For this review, take the finished solid that the model builds, in its own axes (mm). A direction names the side the tool comes from. Coordinates: 2 decimals unless noted, no trailing zeros. Write each loop counter-clockwise with the first axis right and the second up, starting at its lowest first coordinate (ties: lowest second). Pieces come first, ordered by that corner, then holes. Notation, with made-up numbers: (38.25, 73) - (71.25, 73) arc R33 cw to (71.25, 102) - close; hole circle Ø10 at (-31.75, -26.5). An arc over 180 degrees is marked (long way). Write each question's results on one line, items separated by ' | '.
from build123d import *

# Parameters (mm, degrees)
SKETCH_1_W          = 57
SKETCH_1_H          = 37
EXTRUDE_1_DEPTH     = 2
SKETCH_2_W          = 20
SKETCH_2_H          = 2
EXTRUDE_2_DEPTH     = 4
SKETCH_3_R          = 1.05
CUT_EXTRUDE_1_DEPTH = 4
CUT_EXTRUDE_2_DEPTH = 10
FILLET_1_R          = 1.5


with BuildPart() as part:
    # 草图1 → 凸台-拉伸1 (new body)
    with BuildSketch(Plane(origin=(0, 0, 0), x_dir=(1, 0, 0), z_dir=(0, 1, 0))):
        Rectangle(SKETCH_1_W, SKETCH_1_H)
    extrude(amount=EXTRUDE_1_DEPTH)

    # 草图2 → 凸台-拉伸2 (add)
    with BuildSketch(Plane.XY.offset(18.5)):
        with Locations((-3.3, 1)):
            Rectangle(SKETCH_2_W, SKETCH_2_H)
    extrude_2 = extrude(amount=EXTRUDE_2_DEPTH)

    # 镜向1: 凸台-拉伸2 across plane
    add(extrude_2.mirror(Plane.XY))

    # 草图3 → 切除-拉伸1 (cut)
    with BuildSketch(Plane(origin=(0, 2, 0), x_dir=(1, 0, 0), z_dir=(0, 1, 0))):
        with Locations((7.75, 18.5)):
            Circle(SKETCH_3_R)
        with Locations((-14.35, 18.5)):
            Circle(SKETCH_3_R)
        with Locations((-14.35, -18.5)):
            Circle(SKETCH_3_R)
        with Locations((7.75, -18.5)):
            Circle(SKETCH_3_R)
    extrude(amount=-CUT_EXTRUDE_1_DEPTH, mode=Mode.SUBTRACT)

    # 草图4 → 切除-拉伸2 (cut)
    with BuildSketch(Plane(origin=(0, 2, 0), x_dir=(1, 0, 0), z_dir=(0, 1, 0))):
        Polygon((-24.5, -14.5), (-1.963644752, -14.5), (-24.5, 12.175685803), align=None)
        Polygon((-22.536355248, 14.5), (-1.5, -10.400175599), (-1.5, 14.5), align=None)
        Polygon((1.5, 14.5), (1.5, -10.400175599), (22.536355248, 14.5), align=None)
        Polygon((24.5, 12.175685803), (1.963644752, -14.5), (24.5, -14.5), align=None)
    extrude(amount=-CUT_EXTRUDE_2_DEPTH, mode=Mode.SUBTRACT)

    # 圆角1
    fillet_1_edges = [part.edges().sort_by_distance(p)[0] for p in [
        (1.963644752, 1, 14.5),
        (24.5, 1, -12.175685803),
        (24.5, 1, 14.5),
        (-24.5, 1, -12.175685803),
        (-1.963644752, 1, 14.5),
        (-24.5, 1, 14.5),
        (28.5, 1, 18.5),
        (-28.5, 1, 18.5),
        (-28.5, 1, -18.5),
        (28.5, 1, -18.5),
        (-22.536355248, 1, -14.5),
        (-1.5, 1, -14.5),
        (-1.5, 1, 10.400175599),
        (1.5, 1, -14.5),
        (22.536355248, 1, -14.5),
        (1.5, 1, 10.400175599),
    ]]
    fillet(fillet_1_edges, radius=FILLET_1_R)


solid = part.part
Q1. Take a section at B-B on z = 3.5. State the section outline as (x, y) points, plus the area to 3 significant figures.
Results found:
outline: (-28.5, 0) - (-24.5, 0) - (-24.5, 2) - (-28.5, 2) - close; (-11.26, 0) - (-7.33, 0) - (-7.33, 2) - (-11.26, 2) - close; (-1.5, 0) - (1.5, 0) - (1.5, 2) - (-1.5, 2) - close; (7.33, 0) - (11.26, 0) - (11.26, 2) - (7.33, 2) - close; (24.5, 0) - (28.5, 0) - (28.5, 2) - (24.5, 2) - close | area: 37.7 mm2
Q2. Take a section at A-A on x = -12.5. State the section outline as (y, z) points, plus the area to 3 significant figures.
Results found:
outline: (0, -22.5) - (2, -22.5) - (2, -14.5) - (0, -14.5) - close; (0, -2.62) - (2, -2.62) - (2, 2.03) - (0, 2.03) - close; (0, 14.5) - (2, 14.5) - (2, 22.5) - (0, 22.5) - close | area: 41.3 mm2
Q3. For pin 1 (1 mm diameter, centred on x = -21, y = 1, fed in from -Z); pin 2 (0.6 mm diameter, centred on y = 1.5, z = -20, fed in from -X); pin 3 (1 mm diameter, centred on y = 1, z = 20, fed in from +X), all flat-tipped, find the tip position at first contact; note any pin that passes through.
Results found:
pin 1: z = -18.5 | pin 2: x = -13.3 | pin 3: x = 6.7
Q4. Wall thickness on line 1 along Z through (x, y) = (23, 0.9); line 2 along X through (y, z) = (1, -3); line 3 along Z through (x, y) = (-18, 1): over which ranges is each line inside the solid? List them lowest first. Write a range as from..to.
Results found:
line 1: -18.5..-9.58, 14.5..18.5 | line 2: -28.5..-24.5, -16.75..-12.82, -1.5..1.5, 12.82..16.75, 24.5..28.5 | line 3: -18.5..-14.5, -9.13..-4.48, 14.5..18.5
Q5. Take a section at C-C on y = 1.65. State how many separate pieces and enclosed holes the cut face has, plus the area to 3 significant figures.
Results found:
separate pieces: 1 | enclosed holes: 4 | area: 1,160 mm2
Q6. Mouldability with a two-part tool opening along X and no side actions: class faces 1 (the face through (-21, 1, -18.5)), 2 (the face through (14, 1, 14.5)), 3 (the face through (6.7, 1, 20)) as pulls with the +X half, pulls with the -X half, needs draft (parallel to the pull), parting line crosses it, or undercut.
Results found:
face 1: needs draft | face 2: undercut | face 3: pulls with the +X half
Q7. For faces 4 (the face through (-14, 1, 14.5)), 5 (the face through (-13.3, 1, -20)), 6 (the face through (18, 1, -18.5)), list the 3-axis set-ups (+Z, -Z, +X, -X, +Y, -Y) from which the entire face can be reached by the end or side of a thin tool; tool diameter is ignored.
Results found:
face 4: +Y, -Y | face 5: -Z, -X, +Y, -Y | face 6: -Z, +X, +Y, -Y
